Check sheet for the modelled part. Datum: model origin and axes. Units: mm. A direction names the side the tool comes from. Coordinates: 2 decimals unless noted, no trailing zeros. Write each loop counter-clockwise with the first axis right and the second up, starting at its lowest first coordinate (ties: lowest second). Pieces come first, ordered by that corner, then holes. Notation, with made-up numbers: (23, 59.5) - (63, 59.5) arc R26 ccw to (63, 92.5) - close; hole circle Ø10 at (21, 2.25). An arc over 180 degrees is marked (long way). Use one line per item in the form item = value. Start each with the question number.
1. Scan lines: line 1 along Y through (x, z) = (42, 2.65); line 2 along X through (y, z) = (-22, 1.8); line 3 along Y through (x, z) = (84, 1.4). Record each from-to range of solid material in increasing order.
2. Cross-section at A-A on y = 74. Record the boundary of the cut face in (x, z).
3. Cross-section at B-B on x = 133. Record the boundary of the cut face in (y, z), then the cut area to 3 significant figures.
4. Cross-section at D-D on z = 2.2. Give the number of separate pieces and of enclosed holes in the cut face, then the cut area to 3 significant figures.
5. Draft check along Y on faces 1 (the face through (7.804, 113.409, 1.479)), 2 (the face through (162.196, -83.409, 1.479)), 3 (the face through (65.02, 15.88, 1.52)). Enter one of: +Y half, -Y half, draft (parallel to the pull), parting line (faces both ways), or undercut.
6. Tool access check on faces 4 (the face through (112, 17, 0)), 5 (the face through (-13.409, -62.196, 1.479)), 6 (the face through (169.26, -83.3, 1.48)), 7 (the face through (8.175, -83.038, 1.479)), 8 (the face through (183.409, 92.196, 1.479)). Record the directions out of +Z, -Z, +X, -X, +Y, -Y that give a thin tool (end or side, any length) a straight path to the whole face; none if there is none.
7. Go/stop test with flat-tipped pins: pin 1 Ø1.6 at (x, z) = (-25, 1) entering from +Y; pin 2 Ø0.9 at (y, z) = (51.5, 1) entering from +X; pin 3 Ø1.5 at (y, z) = (-27, 1) entering from -X; pin 4 Ø12 at (x, y) = (121.5, 47.5) entering from +Z. Record where each tip stops, or that it passes through.
8. Cross-section at C-C on y = 27. Record the boundary of the cut face in (x, z).
```python
from build123d import *

# Parameters (mm, degrees)
BOSS_EXTRUDE1_DEPTH = 3
SKETCH2_R           = 20
CUT_EXTRUDE1_DEPTH  = 10


with BuildPart() as part:
    # Sketch1 → Boss-Extrude1 (new body)
    with BuildSketch(Plane.XY):
        Polygon((158.754970941, -72.897106565), (180.070576123, -94.00741153), (180.070576123, -95.284756679), (178.131724855, -97.223607947), (175.233947376, -96.447150811), (148.786793436, -69.999996871), (21.213203436, -69.999996871), (-5.233950505, -96.447150811), (-8.131727984, -97.223607947), (-10.070579252, -95.284756679), (-10.070579252, -94.00741153), (11.24502593, -72.897106565), (-2.828675487, -58.686536734), (-24.144280669, -79.796841699), (-25.558494231, -79.796841699), (-27.223611076, -78.131724855), (-26.44715394, -75.233947376), (0, -48.786793435), (0, 78.786796565), (-26.44715394, 105.233950505), (-27.223611076, 108.131727984), (-25.558494231, 109.796844828), (-24.144280669, 109.796844828), (-2.828675487, 88.686539863), (11.24502593, 102.897109694), (-10.070579252, 124.007414659), (-10.070579252, 125.284759808), (-8.131727984, 127.223611076), (-5.233950505, 126.447153941), (21.213203436, 100), (148.786793436, 100), (175.233947376, 126.447153941), (178.131724855, 127.223611076), (180.070576123, 125.284759808), (180.070576123, 124.007414659), (158.754970941, 102.897109694), (172.828672358, 88.686539863), (194.14427754, 109.796844828), (195.558491102, 109.796844828), (197.223607947, 108.131727984), (196.447150812, 105.233950505), (169.999996871, 78.786796565), (169.999996871, -48.786793435), (196.447150812, -75.233947376), (197.223607947, -78.131724855), (195.558491102, -79.796841699), (194.14427754, -79.796841699), (172.828672358, -58.686536734), align=None)
    extrude(amount=BOSS_EXTRUDE1_DEPTH)

    # Sketch2 → Cut-Extrude1 (cut)
    with BuildSketch(Plane.XY.offset(3)):
        with Locations((84.999998436, 15.000001565)):
            Circle(SKETCH2_R)
        Polygon((30, 70), (40, 80), (54.999998436, 80), (54.999998436, 37.500001565), (52.499998436, 35.000001565), (30, 35.000001565), align=None)
        Polygon((30, -4.999998435), (52.499998436, -4.999998435), (54.999998436, -7.499998435), (54.999998436, -49.999996871), (40, -49.999996871), (30, -39.999996871), align=None)
        Polygon((139.999996871, -39.999996871), (139.999996871, -4.999998435), (117.499998436, -4.999998435), (114.999998436, -7.499998435), (114.999998436, -49.999996871), (129.999996871, -49.999996871), align=None)
        Polygon((139.999996871, 35.000001565), (117.499998436, 35.000001565), (114.999998436, 37.500001565), (114.999998436, 80), (129.999996871, 80), (139.999996871, 70), align=None)
    extrude(amount=-CUT_EXTRUDE1_DEPTH, mode=Mode.SUBTRACT)


solid = part.part
```
Final values:
q1.line_1 = -70 to -50, -5 to 35, 80 to 100
q1.line_2 = 0 to 30, 55 to 115, 140 to 170
q1.line_3 = -70 to -4.97, 34.97 to 100
q2.outline = (0, 0) - (34, 0) - (34, 3) - (0, 3) - close; (55, 0) - (115, 0) - (115, 3) - (55, 3) - close; (136, 0) - (170, 0) - (170, 3) - (136, 3) - close
q3.outline = (-70, 0) - (-47, 0) - (-47, 3) - (-70, 3) - close; (-5, 0) - (35, 0) - (35, 3) - (-5, 3) - close; (77, 0) - (100, 0) - (100, 3) - (77, 3) - close
q3.area = 258 mm²
q4.separate_pieces = 1
q4.enclosed_holes = 5
q4.area = 24,800 mm²
q5.face_1 = +Y half
q5.face_2 = -Y half
q5.face_3 = undercut
q6.face_4 = -Z, +X, -X, +Y, -Y
q6.face_5 = +Z, -Z, -X
q6.face_6 = +Z, -Z
q6.face_7 = +Z, -Z, -Y
q6.face_8 = +Z, -Z, +X
q7.pin_1 = 109.8
q7.pin_2 = 170
q7.pin_3 = 0
q7.pin_4 = through
q8.outline = (0, 0) - (69, 0) - (69, 3) - (0, 3) - close; (101, 0) - (170, 0) - (170, 3) - (101, 3) - close
